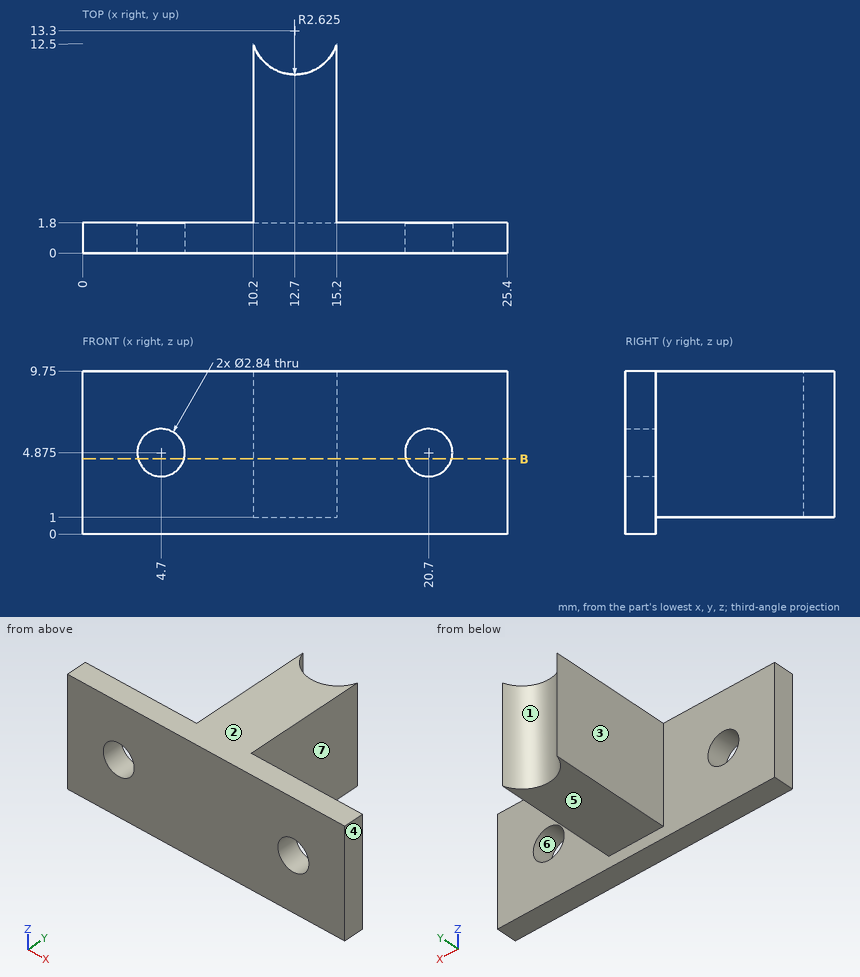
Geometry check sheet. Reference: drawing and pictorial views, mm from the part's lowest x, y, z. A direction names the side the tool comes from. Coordinates: 2 decimals unless noted, no trailing zeros.
Item 1: Depth check by flat-ended pin: pin 1 Ø4.5 at (x, z) = (20.7, 4.875) entering from +Y; pin 2 Ø5 at (x, z) = (10, 2.5) entering from +Y; pin 3 Ø1.5 at (x, y) = (11.5, 6.5) entering from -Z; pin 4 Ø2.5 at (y, z) = (6.5, 5) entering from -X. Enter the tip coordinate at first touch or a pass-through.
Numbers:
pin 1: stops at y = 1.8
pin 2: stops at y = 12.5
pin 3: stops at z = 1
pin 4: stops at x = 10.2
Item 2: Cross-section at B-B on z = 4.5. Count the separate pieces of the cut face and the enclosed holes in it.
Numbers:
separate pieces: 3
enclosed holes: 0
Item 3: Scan lines: probe 1 along X at (y, z) = (10, 2.25); probe 2 along Y at (x, z) = (21.25, 8.75); probe 3 along Z at (x, y) = (12.25, 8.5). Record each from-to range of solid material in increasing order.
Numbers:
probe 1: x = 10.2 to 15.2
probe 2: y = 0 to 1.8
probe 3: z = 1 to 9.75
Item 4: Access from +Z, -Z, +X, -X, +Y, -Y to the whole of each face (thin tool, end or side, straight path). Record for the marked faces 5, 6 and 7.
Numbers:
face 5: -Z, +X, -X, +Y
face 6: +Y, -Y
face 7: +Z, -Z, +X, +Y
Item 5: Mould release check, pull along X, two halves, no side actions. Record for the marked faces 1, 2, 3 and 4: released by +X, released by -X, zero draft, split by the parting line, or undercut.
Numbers:
face 1: undercut
face 2: zero draft
face 3: released by -X
face 4: released by +X
